Here's how the part is built. I have some questions about the finished solid (model axes, mm). Round coordinates to 2 decimals unless told otherwise and drop trailing zeros. Write each loop counter-clockwise with the first axis right and the second up, starting at its lowest first coordinate (ties: lowest second). Pieces come first, ordered by that corner, then holes. Notation, with made-up numbers: (78.25, -7.75) -> (90.25, -7.75) arc R16 ccw to (90.25, 1.25) -> close; hole circle Ø7 at (39, -30.75). An arc over 180 degrees is marked (long way). Answer in a Markdown table with one row per item.
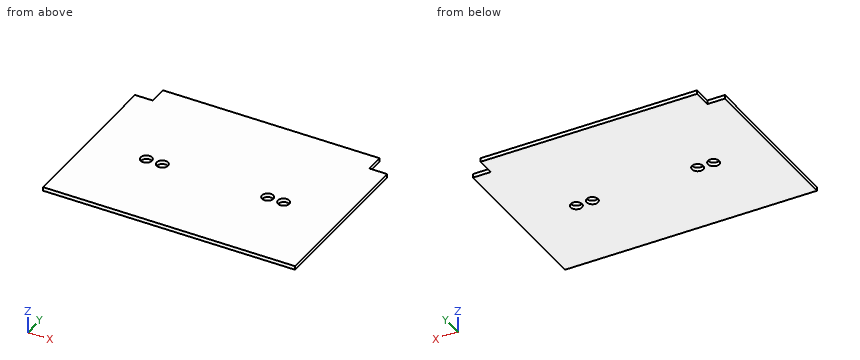
from build123d import *

# Parameters (mm, degrees)
SKETCH1_W           = 400
SKETCH1_H           = 281
BOSS_EXTRUDE1_DEPTH = 6
SKETCH2_W           = 28
SKETCH2_H           = 20
CUT_EXTRUDE1_DEPTH  = 10
SKETCH3_W           = 344
SKETCH3_H           = 9
BOSS_EXTRUDE2_DEPTH = 6
SKETCH4_R           = 9
CUT_EXTRUDE2_DEPTH  = 10


with BuildPart() as part:
    # Sketch1 → Boss-Extrude1 (new body)
    with BuildSketch(Plane.XY):
        with Locations((171.428571429, 117.604761905)):
            Rectangle(SKETCH1_W, SKETCH1_H)
    extrude(amount=BOSS_EXTRUDE1_DEPTH)

    # Sketch2 → Cut-Extrude1 (cut)
    with BuildSketch(Plane.XY.offset(6)):
        with Locations((-14.571428571, 248.104761905)):
            Rectangle(SKETCH2_W, SKETCH2_H)
        with Locations((357.428571429, 248.104761905)):
            Rectangle(SKETCH2_W, SKETCH2_H)
    extrude(amount=-CUT_EXTRUDE1_DEPTH, mode=Mode.SUBTRACT)

    # Sketch3 → Boss-Extrude2 (add)
    with BuildSketch(Plane.XY.offset(6)):
        with Locations((171.428571429, 262.604761905)):
            Rectangle(SKETCH3_W, SKETCH3_H)
    extrude(amount=-BOSS_EXTRUDE2_DEPTH)

    # Sketch4 → Cut-Extrude2 (cut)
    with BuildSketch(Plane.XY.offset(6)):
        with Locations((62.428571429, 107.604761905)):
            Circle(SKETCH4_R)
        with Locations((87.828571429, 107.604761905)):
            Circle(SKETCH4_R)
        with Locations((255.028571429, 107.604761905)):
            Circle(SKETCH4_R)
        with Locations((280.428571429, 107.604761905)):
            Circle(SKETCH4_R)
    extrude(amount=-CUT_EXTRUDE2_DEPTH, mode=Mode.SUBTRACT)


solid = part.part
1) I need wall thicknesses on line 1 (X direction, y = 101, z = 1.35); line 2 (Y direction, x = 96, z = 1.9); line 3 (Y direction, x = 66, z = 1.7). Which ranges of each line are inside material? Lowest first, please. Write a range as [from, to].
Response:
| item | result |
|---|---|
| line 1 | x = [-28.57, 56.31], [68.54, 81.71], [93.94, 248.91], [261.14, 274.31], [286.54, 371.43] |
| line 2 | y = [-22.9, 103.83], [111.38, 267.1] |
| line 3 | y = [-22.9, 99.34], [115.87, 267.1] |
2) I want a section at A-A, the plane x = 87.5. List the corners of the cut face in (y, z) for me, and give its area (3 significant figures).
Response:
| item | result |
|---|---|
| outline | (-22.9, 0) -> (98.61, 0) -> (98.61, 6) -> (-22.9, 6) -> close; (116.6, 0) -> (267.1, 0) -> (267.1, 6) -> (116.6, 6) -> close |
| area | 1,630 mm^2 |
3) For pin 1 (1.8 mm diameter, centred on x = 352.5, z = 2.5, fed in from +Y); pin 2 (1.8 mm diameter, centred on y = 259.5, z = 2.5, fed in from -X); pin 3 (3 mm diameter, centred on y = 253.5, z = 3.5, fed in from +X), each with a flat end and sliding along its axis, tell me the tip position at first contact or that it passes through.
Response:
| item | result |
|---|---|
| pin 1 | stops at y = 238.1 |
| pin 2 | stops at x = -0.57 |
| pin 3 | stops at x = 343.43 |
4) I want a section at B-B, the plane z = 3.9. List the corners of the cut face in (x, y) for me, and give its area (3 significant figures).
Response:
| item | result |
|---|---|
| outline | (-28.57, -22.9) -> (371.43, -22.9) -> (371.43, 238.1) -> (343.43, 238.1) -> (343.43, 267.1) -> (-0.57, 267.1) -> (-0.57, 238.1) -> (-28.57, 238.1) -> close; hole circle Ø18 at (62.43, 107.6); hole circle Ø18 at (87.83, 107.6); hole circle Ø18 at (255.03, 107.6); hole circle Ø18 at (280.43, 107.6) |
| area | 113,000 mm^2 |
5) I want a section at C-C, the plane y = 247. List the corners of the cut face in (x, z) for me.
Response:
| item | result |
|---|---|
| outline | (-0.57, 0) -> (343.43, 0) -> (343.43, 6) -> (-0.57, 6) -> close |
